```python
from build123d import *

# Parameters (mm, degrees)
BOSS_EXTRUDE1_DEPTH = 2
CUT_EXTRUDE1_REACH  = 28.048
SKETCH2_W           = 7
SKETCH2_H           = 17
FILLET1_R           = 2


with BuildPart() as part:
    # Sketch1 → Boss-Extrude1 (new, symmetric)
    with BuildSketch(Plane(origin=(0, 0, 0), x_dir=(1, 0, 0), z_dir=(0, 1, 0))):
        with BuildLine():
            Line((-12.5, -12.5), (12.5, -12.5))
            Line((12.5, -12.5), (12.5, 12.5))
            Line((12.5, 12.5), (1.9814248, 21.752544286))
            ThreePointArc((1.9814248, 21.752544286), (0, 22.5), (-1.9814248, 21.752544286))
            Line((-1.9814248, 21.752544286), (-12.5, 12.5))
            Line((-12.5, 12.5), (-12.5, -12.5))
        make_face()
    extrude(amount=BOSS_EXTRUDE1_DEPTH, both=True)

    # Sketch2 → Cut-Extrude1 (cut, up to next)
    with BuildSketch(Plane(origin=(0, 2, 0), x_dir=(1, 0, 0), z_dir=(0, 1, 0)), mode=Mode.PRIVATE) as cut_extrude1_sk1:
        with Locations((0, -4)):
            Rectangle(SKETCH2_W, SKETCH2_H)
    cut_extrude1_tool1 = extrude(cut_extrude1_sk1.sketch, amount=-CUT_EXTRUDE1_REACH, mode=Mode.PRIVATE) & part.part
    add(cut_extrude1_tool1.solids().sort_by_distance((0, 2, 4))[0], mode=Mode.SUBTRACT)

    # Fillet1
    fillet1_edges = [part.edges().sort_by_distance(p)[0] for p in [
        (-3.5, 0, -4.5),
        (3.5, 0, -4.5),
    ]]
    fillet(fillet1_edges, radius=FILLET1_R)


solid = part.part
```
CAD build for the part. Positions are in the model's coordinates, mm. A direction names the side the tool comes from. Give positions to 0.01 mm unless a question says otherwise; leave off trailing zeros. Order: outer loops, then holes, each group sorted by start corner. A loop starts at its lowest first (then second) coordinate and runs counter-clockwise, first axis right, second up.
(1) Mould opens along X. For faces 3 (the flat face through (0, -2, -5)), 4 (the flat face through (-12.5, 0, 0)), 5 (the flat face through (-3.5, 0, 5)) say: released by +X, released by -X, zero draft, split by the parting line, or undercut.
(2) Flat gauge pins, fed straight in: pin 1 (1.5 mm diameter, centred on x = -0.5, y = -0.5, fed in from +Z); pin 2 (1.5 mm diameter, centred on x = -2, y = -0.5, fed in from +Z). Where does each tip first touch, or does it go through?
(3) Drill centre lines: L1, parallel to X at y = -0.3, z = 6; L2, parallel to Z at x = -0.5, y = -0.3; L3, parallel to Z at x = 2.25, y = 0.9. Where is each one in solid material? Low to high.
(4) Saw through at C-C, the plane z = -3.5. Give the cut face in (x, y), then the cut area to 3 significant figures.
(5) Saw through at B-B, the plane y = -0.95. Give the cut face in (x, z).
(6) Tool access for faces 1 (the flat face through (0, 2, -5)), 2 (the cylindrical face through (-2.93, -0.03, -3.9)): list every direction of +Z, -Z, +X, -X, +Y, -Y with a clear straight run to the whole face (end or side of a thin tool).
(7) Saw through at D-D, the plane x = -5.5. Give the cut face in (y, z).
(8) Saw through at A-A, the plane z = 7. Give the cut face in (x, y), then the cut area to 3 significant figures.
Results found:
1. face 3: zero draft
1. face 4: released by -X
1. face 5: undercut
2. pin 1: stops at z = -4.5
2. pin 2: stops at z = -4.06
3. L1: x = -12.5 to -3.5, 3.5 to 12.5
3. L2: z = -22.46 to -4.5
3. L3: z = -21.52 to -4.35
4. outline: (-12.5, -2) - (-3.23, -2) - (-3.23, 2) - (-12.5, 2) - close; (3.23, -2) - (12.5, -2) - (12.5, 2) - (3.23, 2) - close
4. area: 74.1 mm2
5. outline: (-12.5, -12.5) - (-1.98, -21.75) arc R3 ccw to (1.98, -21.75) - (12.5, -12.5) - (12.5, 12.5) - (3.5, 12.5) - (3.5, -2.5) arc R2 cw to (1.5, -4.5) - (-1.5, -4.5) arc R2 cw to (-3.5, -2.5) - (-3.5, 12.5) - (-12.5, 12.5) - close
6. face 1: +Z, -Z, +X, -X, +Y
6. face 2: +Z, +Y, -Y
7. outline: (-2, -18.66) - (2, -18.66) - (2, 12.5) - (-2, 12.5) - close
8. outline: (-12.5, -2) - (-3.5, -2) - (-3.5, 2) - (-12.5, 2) - close; (3.5, -2) - (12.5, -2) - (12.5, 2) - (3.5, 2) - close
8. area: 72.0 mm2
